Autodesk Inventor part; units mm, degrees
ref_plane "YZ Plane" through (0, 0, 0) normal (1, 0, 0) x (0, 1, 0)
ref_plane "XZ Plane" through (0, 0, 0) normal (0, 1, 0) x (-1, 0, 0)
ref_plane "XY Plane" through (0, 0, 0) normal (0, 0, 1) x (1, 0, 0)
sketch "Sketch1" plane through (0, 0, 0) normal (0, 1, 0) x (-1, 0, 0)
  line L0 (20.25, -10) -> (-20.25, -10)
  line L1 (-20.25, -10) -> (-20.25, 10)
  line L2 (-20.25, 10) -> (20.25, 10)
  line L3 (20.25, 10) -> (20.25, -10)
  point P0 (0, 0)
  dimension "d0" = 40.5
  dimension "d1" = 20
  dimension "d2" = 10
  dimension "d3" = 20.25
extrude "Plate1" add sketch "Sketch1" along normal blind 1.5
sketch "Sketch2" plane through (21.75, 0, -10) normal (-1, 0, 0) x (0, -1, 0)
  line L0 (0, 20) -> (0, 0)
  line L1 (0, 0) -> (-45, 0)
  line L2 (-45, 0) -> (-45, 20)
  line L3 (-45, 20) -> (0, 20)
edge flange "Flange1" height 45 angle 90 thickness 1.5 bend radius 0.31 thickness toward (-1, 0, 0) relief tear relief width 1.5 relief depth 0.75 edges at (20.25, 1.5, 0) wall of the first edge with corners at (21.75, 0, 10) (21.75, 0, -10) (21.75, 45, -10) (21.75, 45, 10)
bend "Bend1"
corner "Corner1"
sketch "Sketch3" plane through (-21.75, 0, 10) normal (1, 0, 0) x (0, 1, 0)
  line L0 (0, -20) -> (0, 0)
  line L1 (0, 0) -> (45, 0)
  line L2 (45, 0) -> (45, -20)
  line L3 (45, -20) -> (0, -20)
edge flange "Flange2" height 45 angle 90 thickness 1.5 bend radius 0.31 thickness toward (1, 0, 0) relief tear relief width 1.5 relief depth 0.75 edges at (-20.25, 1.5, 0) wall of the first edge with corners at (-21.75, 0, -10) (-21.75, 0, 10) (-21.75, 45, 10) (-21.75, 45, -10)
bend "Bend2"
corner "Corner2"
sketch "Sketch4" plane through (21.75, 45, 10) normal (1, 0, 0) x (0, 0, -1)
  circle A0 centre (10, -9.9) radius 6.4
  line L0 (0, 0) -> (20, 0)
  line L1 (20, 0) -> (20, -43.19)
  point P0 (10, -45)
  dimension "d25" = 9.9
  dimension "d26" = 12.8
  dimension "d27" = 10
extrude "Extrusion1" cut sketch "Sketch4" against normal blind 50
sketch "Sketch5" plane through (21.75, 45, 10) normal (1, 0, 0) x (0, 0, -1)
  circle A0 centre (10, -9.9) radius 6.4
  line L0 (0, 0) -> (20, 0)
  line L1 (-4, 0) -> (24, 0)
  line L2 (24, 0) -> (24, -9.9)
  line L3 (24, -9.9) -> (-4, -9.9)
  line L4 (-4, -9.9) -> (-4, 0)
  line L5 (0, -43.19) -> (0, 0)
  point P0 (10, -45)
  dimension "d30" = 9.9
  dimension "d31" = 28
  dimension "d32" = 4
extrude "Extrusion2" cut sketch "Sketch5" against normal blind 50 contours L3 A0 | A0 L3 L5 L0 L1 L2 | L3 L4 L1 L5 picked at (9.2435, -7.9053)
fillet "Fillet1" radius 1 4 edges at (-21, 35.1, 10) (-21, 35.1, -10) (21, 35.1, -10) (21, 35.1, 10)
sketch "Sketch8" plane through (0, 0, 0) normal (0, -1, 0) x (1, 0, 0)
  circle A0 centre (8, -8) radius 1.05
  circle A1 centre (-8, -8) radius 1.05
  circle A2 centre (8, 8) radius 1.05
  circle A3 centre (-8, 8) radius 1.05
  point P0 (0, 0)
hole "Hole3" at (8, 0, -8) at (-8, 0, -8) at (-8, 0, 8) at (8, 0, 8) direction (0, 1, 0) diameter 2.1 depth 1.5
equation "\"d55\" = Thickness"
equation "\"d4\" = Thickness"
equation "\"d5\" = BendReliefWidth"
equation "\"d6\" = BendReliefDepth"
equation "\"d7\" = MinimumRemnant"
equation "\"d8\" = TransitionRadius"
equation "\"d11\" = BendRadius"
equation "\"d12\" = CornerReliefSize"
equation "\"d13\" = GapSize"
equation "\"d14\" = JacobiRadiusSize"
equation "\"d15\" = BendReliefWidth"
equation "\"d16\" = BendReliefDepth"
equation "\"d17\" = MinimumRemnant"
equation "\"d18\" = TransitionRadius"
equation "\"d21\" = BendRadius"
equation "\"d22\" = CornerReliefSize"
equation "\"d23\" = GapSize"
equation "\"d24\" = JacobiRadiusSize"
equation "\"BendReliefWidth\" = Thickness"
equation "\"BendReliefDepth\" = 0.5 * Thickness"
equation "\"CornerReliefSize\" = 4 * Thickness"
equation "\"MinimumRemnant\" = 2 * Thickness"
equation "\"TransitionRadius\" = BendRadius"
equation "\"JacobiRadiusSize\" = BendRadius"
equation "\"GapSize\" = Thickness"
properties part number "axis_10_top_frame" material "Aluminum 6061-AHC"
Work out the finished part from the listing and answer in its coordinate system (mm). A direction names the side the tool comes from. Round coordinates to 2 decimals unless told otherwise and drop trailing zeros. Write each loop counter-clockwise with the first axis right and the second up, starting at its lowest first coordinate (ties: lowest second). Pieces come first, ordered by that corner, then holes. Notation, with made-up numbers: (8.5, 22.5) -> (42.5, 22.5) arc R37 cw to (42.5, 59.5) -> close; hole circle Ø2 at (-25.5, 82). An arc over 180 degrees is marked (long way). Write each question's results on one line, items separated by ' | '.
Item 1: Find the intervals of material crossed by line 1 along Z through (x, y) = (8, 0.3); line 2 along X through (y, z) = (17, 3.5); line 3 along X through (y, z) = (0.55, 8), in increasing order. Write a range as [from, to].
Result set:
line 1: [-10, -9.05], [-6.95, 6.95], [9.05, 10] | line 2: [-21.75, -20.25], [20.25, 21.75] | line 3: [-21.24, -9.05], [-6.95, 6.95], [9.05, 21.24]
Item 2: A cutting plane is placed at C-C, the plane y = 23. Determine the outline of the cut face in (x, z).
Result set:
outline: (-21.75, -10) -> (-20.25, -10) -> (-20.25, 10) -> (-21.75, 10) -> close; (20.25, -10) -> (21.75, -10) -> (21.75, 10) -> (20.25, 10) -> close
Item 3: A cutting plane is placed at B-B, the plane z = -8. Determine the outline of the cut face in (x, y).
Result set:
outline: (-21.75, 1.81) arc R1.81 ccw to (-19.94, 0) -> (-9.05, 0) -> (-9.05, 1.5) -> (-19.94, 1.5) arc R0.31 cw to (-20.25, 1.81) -> (-20.25, 35.1) -> (-21.75, 35.1) -> close; (-6.95, 0) -> (6.95, 0) -> (6.95, 1.5) -> (-6.95, 1.5) -> close; (9.05, 0) -> (19.94, 0) arc R1.81 ccw to (21.75, 1.81) -> (21.75, 35.1) -> (20.25, 35.1) -> (20.25, 1.81) arc R0.31 cw to (19.94, 1.5) -> (9.05, 1.5) -> close
Item 4: Which of the six approach directions +Z, -Z, +X, -X, +Y, -Y give full straight-line access (tool end or side, diameter ignored) to faces 4 (the face through (20.99, 34.799, 9.715)), 5 (the face through (0, 1.5, 0))?
Result set:
face 4: +Z, +X, -X, +Y | face 5: +Z, -Z, +Y
Item 5: The mould has two halves that part along X. Classify faces 1 (the face through (21.75, 19, 0)), 2 (the face through (-9.04, 0.76, -7.86)), 3 (the face through (0, 0, 0)): +X half, -X half, draft (parallel to the pull), parting line (faces both ways), or undercut.
Result set:
face 1: +X half | face 2: undercut | face 3: draft
Item 6: A cutting plane is placed at A-A, the plane x = -8. Determine the outline of the cut face in (y, z), plus the area to 3 significant figures.
Result set:
outline: (0, -10) -> (1.5, -10) -> (1.5, -9.05) -> (0, -9.05) -> close; (0, -6.95) -> (1.5, -6.95) -> (1.5, 6.95) -> (0, 6.95) -> close; (0, 9.05) -> (1.5, 9.05) -> (1.5, 10) -> (0, 10) -> close | area: 23.7 mm^2
Item 7: A cutting plane is placed at D-D, the plane z = 0. Determine the outline of the cut face in (x, y).
Result set:
outline: (-21.75, 1.81) arc R1.81 ccw to (-19.94, 0) -> (19.94, 0) arc R1.81 ccw to (21.75, 1.81) -> (21.75, 28.7) -> (20.25, 28.7) -> (20.25, 1.81) arc R0.31 cw to (19.94, 1.5) -> (-19.94, 1.5) arc R0.31 cw to (-20.25, 1.81) -> (-20.25, 28.7) -> (-21.75, 28.7) -> close
Item 8: A flat-ended cylindrical pin translates along its axis: P1, Ø1.5, axis at x = -2, z = -3, coming from the +Y side. Find the tip coordinate at first contact, or state that the pin passes through.
Result set:
P1: y = 1.5
